Input: part model. Units: mm. Frame: model coordinates. Coordinates: 2 decimals unless noted, no trailing zeros. Loops run counter-clockwise (first coordinate to the right, second up) from the corner with the lowest first, then second, coordinate; pieces in that order, holes last. Notation, with made-up numbers: (89.5, -26) - (131.5, -26) arc R26 cw to (131.5, -11) - close; hole circle Ø7 at (79.5, 80). An arc over 180 degrees is marked (long way). Use a Markdown table: item, result. Add a question column.
1. Section query C-C on z = -2. Return the cut outline in (x, y) (3 decimals), then the cut area to 3 significant figures.
2. Section query B-B on z = -19.05. State how many separate pieces and enclosed holes the cut face has, then the cut area to 3 significant figures.
3. Ray query, L1, parallel to Z at x = -1, y = 2.5; L2, parallel to Z at x = -3.5, y = 2.45. Return the intervals inside material, ascending. Write a range as [from, to].
4. Section query A-A on x = -2.5. Return the cut outline in (y, z) (3 decimals), then the cut area to 3 significant figures.
```python
from build123d import *

# Parameters (mm, degrees)
SKETCH1_W           = 127
SKETCH1_H           = 127
SKETCH1_R           = 5.272810933
SKETCH1_R_2         = 4.510308164
SKETCH1_R_3         = 3.429
BOSS_EXTRUDE1_DEPTH = 3.175


with BuildPart() as part:
    # Sketch1 → Boss-Extrude1 (new body)
    with BuildSketch(Plane(origin=(0, 0, 0), x_dir=(1, 0, 0), z_dir=(0, 1, 0))):
        Rectangle(SKETCH1_W, SKETCH1_H)
        with Locations(Location((0, 19.05, 0), (0, 0, 270))):
            Circle(SKETCH1_R, mode=Mode.SUBTRACT)
        with Locations(Location((0, 57.15, 0), (0, 0, 270))):
            Circle(SKETCH1_R_2, mode=Mode.SUBTRACT)
        with Locations(Location((57.15, 0, 0), (0, 0, 90))):
            Circle(SKETCH1_R_2, mode=Mode.SUBTRACT)
        with Locations(Location((19.05, 0, 0), (0, 0, 90))):
            Circle(SKETCH1_R, mode=Mode.SUBTRACT)
        with Locations(Location((0, -19.05, 0), (0, 0, 270))):
            Circle(SKETCH1_R, mode=Mode.SUBTRACT)
        with Locations(Location((0, -57.15, 0), (0, 0, 270))):
            Circle(SKETCH1_R_2, mode=Mode.SUBTRACT)
        with Locations(Location((-57.15, 0, 0), (0, 0, 90))):
            Circle(SKETCH1_R_2, mode=Mode.SUBTRACT)
        with Locations(Location((-19.05, 0, 0), (0, 0, 90))):
            Circle(SKETCH1_R, mode=Mode.SUBTRACT)
        with Locations(Location((-57.15, 57.15, 0), (0, 0, 270))):
            Circle(SKETCH1_R_3, mode=Mode.SUBTRACT)
        with Locations(Location((-44.45, 57.15, 0), (0, 0, 270))):
            Circle(SKETCH1_R_3, mode=Mode.SUBTRACT)
        with Locations(Location((-31.75, 57.15, 0), (0, 0, 270))):
            Circle(SKETCH1_R_3, mode=Mode.SUBTRACT)
        with Locations(Location((-19.05, 57.15, 0), (0, 0, 270))):
            Circle(SKETCH1_R_3, mode=Mode.SUBTRACT)
        with Locations(Location((19.05, 57.15, 0), (0, 0, 270))):
            Circle(SKETCH1_R_3, mode=Mode.SUBTRACT)
        with Locations(Location((31.75, 57.15, 0), (0, 0, 270))):
            Circle(SKETCH1_R_3, mode=Mode.SUBTRACT)
        with Locations(Location((44.45, 57.15, 0), (0, 0, 270))):
            Circle(SKETCH1_R_3, mode=Mode.SUBTRACT)
        with Locations(Location((57.15, 57.15, 0), (0, 0, 270))):
            Circle(SKETCH1_R_3, mode=Mode.SUBTRACT)
        with Locations(Location((-44.45, 44.45, 0), (0, 0, 270))):
            Circle(SKETCH1_R_3, mode=Mode.SUBTRACT)
        with Locations(Location((-31.75, 44.45, 0), (0, 0, 270))):
            Circle(SKETCH1_R_3, mode=Mode.SUBTRACT)
        with Locations(Location((-19.05, 44.45, 0), (0, 0, 270))):
            Circle(SKETCH1_R_3, mode=Mode.SUBTRACT)
        with Locations(Location((19.05, 44.45, 0), (0, 0, 270))):
            Circle(SKETCH1_R_3, mode=Mode.SUBTRACT)
        with Locations(Location((31.75, 44.45, 0), (0, 0, 270))):
            Circle(SKETCH1_R_3, mode=Mode.SUBTRACT)
        with Locations(Location((44.45, 44.45, 0), (0, 0, 270))):
            Circle(SKETCH1_R_3, mode=Mode.SUBTRACT)
        with Locations(Location((57.15, 44.45, 0), (0, 0, 270))):
            Circle(SKETCH1_R_3, mode=Mode.SUBTRACT)
        with Locations(Location((-44.45, 31.75, 0), (0, 0, 270))):
            Circle(SKETCH1_R_3, mode=Mode.SUBTRACT)
        with Locations(Location((-31.75, 31.75, 0), (0, 0, 270))):
            Circle(SKETCH1_R_3, mode=Mode.SUBTRACT)
        with Locations(Location((-19.05, 31.75, 0), (0, 0, 270))):
            Circle(SKETCH1_R_3, mode=Mode.SUBTRACT)
        with Locations(Location((19.05, 31.75, 0), (0, 0, 270))):
            Circle(SKETCH1_R_3, mode=Mode.SUBTRACT)
        with Locations(Location((31.75, 31.75, 0), (0, 0, 270))):
            Circle(SKETCH1_R_3, mode=Mode.SUBTRACT)
        with Locations(Location((44.45, 31.75, 0), (0, 0, 270))):
            Circle(SKETCH1_R_3, mode=Mode.SUBTRACT)
        with Locations(Location((57.15, 31.75, 0), (0, 0, 270))):
            Circle(SKETCH1_R_3, mode=Mode.SUBTRACT)
        with Locations(Location((-44.45, 19.05, 0), (0, 0, 270))):
            Circle(SKETCH1_R_3, mode=Mode.SUBTRACT)
        with Locations(Location((-31.75, 19.05, 0), (0, 0, 270))):
            Circle(SKETCH1_R_3, mode=Mode.SUBTRACT)
        with Locations(Location((-19.05, 19.05, 0), (0, 0, 270))):
            Circle(SKETCH1_R_3, mode=Mode.SUBTRACT)
        with Locations(Location((19.05, 19.05, 0), (0, 0, 270))):
            Circle(SKETCH1_R_3, mode=Mode.SUBTRACT)
        with Locations(Location((31.75, 19.05, 0), (0, 0, 270))):
            Circle(SKETCH1_R_3, mode=Mode.SUBTRACT)
        with Locations(Location((44.45, 19.05, 0), (0, 0, 270))):
            Circle(SKETCH1_R_3, mode=Mode.SUBTRACT)
        with Locations(Location((57.15, 19.05, 0), (0, 0, 270))):
            Circle(SKETCH1_R_3, mode=Mode.SUBTRACT)
        with Locations(Location((-44.45, -19.05, 0), (0, 0, 270))):
            Circle(SKETCH1_R_3, mode=Mode.SUBTRACT)
        with Locations(Location((-31.75, -19.05, 0), (0, 0, 270))):
            Circle(SKETCH1_R_3, mode=Mode.SUBTRACT)
        with Locations(Location((-19.05, -19.05, 0), (0, 0, 270))):
            Circle(SKETCH1_R_3, mode=Mode.SUBTRACT)
        with Locations(Location((19.05, -19.05, 0), (0, 0, 270))):
            Circle(SKETCH1_R_3, mode=Mode.SUBTRACT)
        with Locations(Location((31.75, -19.05, 0), (0, 0, 270))):
            Circle(SKETCH1_R_3, mode=Mode.SUBTRACT)
        with Locations(Location((44.45, -19.05, 0), (0, 0, 270))):
            Circle(SKETCH1_R_3, mode=Mode.SUBTRACT)
        with Locations(Location((57.15, -19.05, 0), (0, 0, 270))):
            Circle(SKETCH1_R_3, mode=Mode.SUBTRACT)
        with Locations(Location((-44.45, -31.75, 0), (0, 0, 270))):
            Circle(SKETCH1_R_3, mode=Mode.SUBTRACT)
        with Locations(Location((-31.75, -31.75, 0), (0, 0, 270))):
            Circle(SKETCH1_R_3, mode=Mode.SUBTRACT)
        with Locations(Location((-19.05, -31.75, 0), (0, 0, 270))):
            Circle(SKETCH1_R_3, mode=Mode.SUBTRACT)
        with Locations(Location((19.05, -31.75, 0), (0, 0, 270))):
            Circle(SKETCH1_R_3, mode=Mode.SUBTRACT)
        with Locations(Location((31.75, -31.75, 0), (0, 0, 270))):
            Circle(SKETCH1_R_3, mode=Mode.SUBTRACT)
        with Locations(Location((44.45, -31.75, 0), (0, 0, 270))):
            Circle(SKETCH1_R_3, mode=Mode.SUBTRACT)
        with Locations(Location((57.15, -31.75, 0), (0, 0, 270))):
            Circle(SKETCH1_R_3, mode=Mode.SUBTRACT)
        with Locations(Location((-44.45, -44.45, 0), (0, 0, 270))):
            Circle(SKETCH1_R_3, mode=Mode.SUBTRACT)
        with Locations(Location((-31.75, -44.45, 0), (0, 0, 270))):
            Circle(SKETCH1_R_3, mode=Mode.SUBTRACT)
        with Locations(Location((-19.05, -44.45, 0), (0, 0, 270))):
            Circle(SKETCH1_R_3, mode=Mode.SUBTRACT)
        with Locations(Location((19.05, -44.45, 0), (0, 0, 270))):
            Circle(SKETCH1_R_3, mode=Mode.SUBTRACT)
        with Locations(Location((31.75, -44.45, 0), (0, 0, 270))):
            Circle(SKETCH1_R_3, mode=Mode.SUBTRACT)
        with Locations(Location((44.45, -44.45, 0), (0, 0, 270))):
            Circle(SKETCH1_R_3, mode=Mode.SUBTRACT)
        with Locations(Location((57.15, -44.45, 0), (0, 0, 270))):
            Circle(SKETCH1_R_3, mode=Mode.SUBTRACT)
        with Locations(Location((-44.45, -57.15, 0), (0, 0, 270))):
            Circle(SKETCH1_R_3, mode=Mode.SUBTRACT)
        with Locations(Location((-31.75, -57.15, 0), (0, 0, 270))):
            Circle(SKETCH1_R_3, mode=Mode.SUBTRACT)
        with Locations(Location((-19.05, -57.15, 0), (0, 0, 270))):
            Circle(SKETCH1_R_3, mode=Mode.SUBTRACT)
        with Locations(Location((19.05, -57.15, 0), (0, 0, 270))):
            Circle(SKETCH1_R_3, mode=Mode.SUBTRACT)
        with Locations(Location((31.75, -57.15, 0), (0, 0, 270))):
            Circle(SKETCH1_R_3, mode=Mode.SUBTRACT)
        with Locations(Location((44.45, -57.15, 0), (0, 0, 270))):
            Circle(SKETCH1_R_3, mode=Mode.SUBTRACT)
        with Locations(Location((57.15, -57.15, 0), (0, 0, 270))):
            Circle(SKETCH1_R_3, mode=Mode.SUBTRACT)
        with Locations(Location((-57.15, 44.45, 0), (0, 0, 270))):
            Circle(SKETCH1_R_3, mode=Mode.SUBTRACT)
        with Locations(Location((-57.15, 31.75, 0), (0, 0, 270))):
            Circle(SKETCH1_R_3, mode=Mode.SUBTRACT)
        with Locations(Location((-57.15, 19.05, 0), (0, 0, 270))):
            Circle(SKETCH1_R_3, mode=Mode.SUBTRACT)
        with Locations(Location((-57.15, -19.05, 0), (0, 0, 270))):
            Circle(SKETCH1_R_3, mode=Mode.SUBTRACT)
        with Locations(Location((-57.15, -31.75, 0), (0, 0, 270))):
            Circle(SKETCH1_R_3, mode=Mode.SUBTRACT)
        with Locations(Location((-57.15, -44.45, 0), (0, 0, 270))):
            Circle(SKETCH1_R_3, mode=Mode.SUBTRACT)
        with Locations(Location((-57.15, -57.15, 0), (0, 0, 270))):
            Circle(SKETCH1_R_3, mode=Mode.SUBTRACT)
    extrude(amount=BOSS_EXTRUDE1_DEPTH)


solid = part.part
```
Resolved:
| question | item | result |
|---|---|---|
| 1 | outline | (-63.5, 0) - (-61.193, 0) - (-61.193, 3.175) - (-63.5, 3.175) - close; (-53.107, 0) - (-23.929, 0) - (-23.929, 3.175) - (-53.107, 3.175) - close; (-14.171, 0) - (14.171, 0) - (14.171, 3.175) - (-14.171, 3.175) - close; (23.929, 0) - (53.107, 0) - (53.107, 3.175) - (23.929, 3.175) - close; (61.193, 0) - (63.5, 0) - (63.5, 3.175) - (61.193, 3.175) - close |
| 1 | area | 290 mm² |
| 2 | separate pieces | 10 |
| 2 | enclosed holes | 0 |
| 2 | area | 196 mm² |
| 3 | L1 | [-63.5, -61.55], [-52.75, -24.23], [-13.87, 13.87], [24.23, 52.75], [61.55, 63.5] |
| 3 | L2 | [-63.5, -59.99], [-54.31, -22.99], [-15.11, 15.11], [22.99, 54.31], [59.99, 63.5] |
| 4 | outline | (0, -63.5) - (3.175, -63.5) - (3.175, -60.904) - (0, -60.904) - close; (0, -53.396) - (3.175, -53.396) - (3.175, -23.692) - (0, -23.692) - close; (0, -14.408) - (3.175, -14.408) - (3.175, 14.408) - (0, 14.408) - close; (0, 23.692) - (3.175, 23.692) - (3.175, 53.396) - (0, 53.396) - close; (0, 60.904) - (3.175, 60.904) - (3.175, 63.5) - (0, 63.5) - close |
| 4 | area | 297 mm² |
